from build123d import *

# Parameters (mm, degrees)
EXTRUDE4_DEPTH          = 1.9304
SKETCH2_R               = 0.6604
CUT_EXTRUDE1_DEPTH      = 19.722050478
CIRPATTERN4_COUNT       = 6
CUT_EXTRUDE2_DEPTH      = 12.7
CUT_EXTRUDE2_DEPTH_BACK = 12.7
SKETCH3_R               = 1.397
SKETCH4_R               = 4.445
CUT_EXTRUDE3_DEPTH      = 0.635
SKETCH5_R               = 3.4925
SKETCH5_R_2             = 3.175
EXTRUDE5_DEPTH          = 1.143
RIB10_REACH             = 26.438
SKETCH8_WALL_W          = 52.220152264
SKETCH8_WALL_H          = 0.381
CIRPATTERN5_COUNT       = 8
SKETCH9_R               = 0.79375
SKETCH9_R_2             = 1.1938
CUT_EXTRUDE4_DEPTH      = 25.392925761
CIRPATTERN6_COUNT       = 6
SKETCH10_R              = 5.08
EXTRUDE6_DEPTH          = 0.762
FILLET2_R               = 0.508
SKETCH11_R              = 4.064
EXTRUDE7_DEPTH          = 3.048
FILLET3_R               = 0.889
SKETCH12_R              = 2.8575
CUT_EXTRUDE5_DEPTH      = 3.429
SKETCH14_R              = 1.397
CUT_EXTRUDE6_DEPTH      = 25.557003564
SKETCH15_R              = 0.3175
CUT_EXTRUDE7_DEPTH      = 25.984806887
CIRPATTERN7_COUNT       = 6


with BuildPart() as part:
    # Sketch1 → Extrude4 (new body)
    with BuildSketch(Plane(origin=(0, 0, 0), x_dir=(1, 0, 0), z_dir=(0, 1, 0))):
        with BuildLine():
            Line((5.775220615, -3.829827046), (0, 0))
            Line((0, 0), (5.775220615, 3.829827046))
            Line((5.775220615, 3.829827046), (6.35029977, 3.829827046))
            Line((6.35029977, 3.829827046), (6.35029977, 3.494998084))
            Line((6.35029977, 3.494998084), (15.87469147, 2.35207108))
            ThreePointArc((15.87469147, 2.35207108), (18.22419147, 0.00257108), (15.87469147, -2.34692892))
            Line((15.87469147, -2.34692892), (6.34969147, -3.48992892))
            Line((6.34969147, -3.48992892), (6.34969147, -3.829827046))
            Line((6.34969147, -3.829827046), (5.775220615, -3.829827046))
        make_face()
    extrude4 = extrude(amount=EXTRUDE4_DEPTH)

    # Sketch2 → Cut-Extrude1 (cut, through all)
    with BuildSketch(Plane(origin=(0, 1.9304, 0), x_dir=(-1, 0, 0), z_dir=(0, 1, 0))):
        with Locations((-6.342552501, -4.149920748)):
            Circle(SKETCH2_R)
        with Locations((-6.342552501, 4.149920748)):
            Circle(SKETCH2_R)
    extrude(amount=-CUT_EXTRUDE1_DEPTH, mode=Mode.SUBTRACT)

    # CirPattern4: Extrude4 ×6 about axis
    cirpattern4_axis = Axis((0, 0, 0), (0, 1, 0))
    for i in range(1, CIRPATTERN4_COUNT):
        add(extrude4.rotate(cirpattern4_axis, i * 360 / CIRPATTERN4_COUNT))

    # Sketch3 → Cut-Extrude2 (cut, two sides: drawn at the far end of the back side and taken through both)
    with BuildSketch(Plane(origin=(0, 1.9304, 0), x_dir=(-1, 0, 0), z_dir=(0, 1, 0)).offset(-CUT_EXTRUDE2_DEPTH_BACK)):
        with Locations(Location((0, 0, 0), (0, 0, 90))):
            Circle(SKETCH3_R)
    extrude(amount=CUT_EXTRUDE2_DEPTH + CUT_EXTRUDE2_DEPTH_BACK, mode=Mode.SUBTRACT)

    # Sketch4 → Cut-Extrude3 (cut)
    with BuildSketch(Plane(origin=(0, 1.9304, 0), x_dir=(-1, 0, 0), z_dir=(0, 1, 0))):
        with Locations(Location((0, 0, 0), (0, 0, 90))):
            Circle(SKETCH4_R)
    extrude(amount=-CUT_EXTRUDE3_DEPTH, mode=Mode.SUBTRACT)

    # Sketch5 → Extrude5 (add)
    with BuildSketch(Plane(origin=(0, 1.2954, 0), x_dir=(-1, 0, 0), z_dir=(0, 1, 0))):
        with Locations(Location((0, 0, 0), (0, 0, 90))):
            Circle(SKETCH5_R)
        with Locations(Location((0, 0, 0), (0, 0, 90))):
            Circle(SKETCH5_R_2, mode=Mode.SUBTRACT)
    extrude(amount=EXTRUDE5_DEPTH)

    # Sketch8 wall → Rib10 (add, up to next)
    with BuildSketch(Plane(origin=(-3.967749561, 1.770078976, 0), x_dir=(-0.70753138537, -0.706681921883, 0), z_dir=(0.706681921883, -0.70753138537, 0)), mode=Mode.PRIVATE) as rib10_sk1:
        Rectangle(SKETCH8_WALL_W, SKETCH8_WALL_H)
    rib10_tool1 = extrude(rib10_sk1.sketch, amount=RIB10_REACH, mode=Mode.PRIVATE) - part.part
    rib10 = rib10_tool1.solids().sort_by_distance((-3.967749561, 1.770078976, 0))[0]
    add(rib10)

    # CirPattern5: Rib10 ×8 about axis
    cirpattern5_axis = Axis((0, 0, 0), (0, 1, 0))
    for i in range(1, CIRPATTERN5_COUNT):
        add(rib10.rotate(cirpattern5_axis, i * 360 / CIRPATTERN5_COUNT))

    # Sketch9 → Cut-Extrude4 (cut, through all)
    with BuildSketch(Plane(origin=(0, 1.9304, 0), x_dir=(-1, 0, 0), z_dir=(0, 1, 0))):
        with Locations(Location((7.935119114, 13.749171631, 0), (0, 0, 90))):
            Circle(SKETCH9_R)
        with Locations(Location((5.256324989, 9.107628175, 0), (0, 0, 90))):
            Circle(SKETCH9_R_2)
    cut_extrude4 = extrude(amount=-CUT_EXTRUDE4_DEPTH, mode=Mode.SUBTRACT)

    # CirPattern6: Cut-Extrude4 ×6 about axis
    cirpattern6_axis = Axis((0, 0, 0), (0, 1, 0))
    for i in range(1, CIRPATTERN6_COUNT):
        add(cut_extrude4.rotate(cirpattern6_axis, i * 360 / CIRPATTERN6_COUNT), mode=Mode.SUBTRACT)

    # Sketch10 → Extrude6 (add)
    with BuildSketch(Plane.XZ):
        with Locations(Location((0, 0, 0), (0, 0, 90))):
            Circle(SKETCH10_R)
    extrude(amount=EXTRUDE6_DEPTH)

    # Fillet2
    fillet2_edges = [part.edges().sort_by_distance(p)[0] for p in [
        (0, 0, -5.08),
    ]]
    fillet(fillet2_edges, radius=FILLET2_R)

    # Sketch11 → Extrude7 (add)
    with BuildSketch(Plane.XZ.offset(0.762)):
        with Locations(Location((0, 0, 0), (0, 0, 90))):
            Circle(SKETCH11_R)
    extrude(amount=EXTRUDE7_DEPTH)

    # Fillet3
    fillet3_edges = [part.edges().sort_by_distance(p)[0] for p in [
        (0, -0.762, -4.064),
    ]]
    fillet(fillet3_edges, radius=FILLET3_R)

    # Sketch12 → Cut-Extrude5 (cut)
    with BuildSketch(Plane.XZ.offset(3.81)):
        with Locations(Location((0, 0, 0), (0, 0, 270))):
            Circle(SKETCH12_R)
    extrude(amount=-CUT_EXTRUDE5_DEPTH, mode=Mode.SUBTRACT)

    # Sketch14 → Cut-Extrude6 (cut, through all)
    with BuildSketch(Plane.XZ.offset(0.381)):
        with Locations(Location((0, 0, 0), (0, 0, 90))):
            Circle(SKETCH14_R)
    extrude(amount=-CUT_EXTRUDE6_DEPTH, mode=Mode.SUBTRACT)

    # Sketch15 → Cut-Extrude7 (cut, symmetric)
    with BuildSketch(Plane(origin=(0, 1.9304, 0), x_dir=(-1, 0, 0), z_dir=(0, 1, 0))):
        with Locations((-6.48724684, -3.751940905)):
            Circle(SKETCH15_R)
    cut_extrude7 = extrude(amount=CUT_EXTRUDE7_DEPTH, both=True, mode=Mode.SUBTRACT)

    # CirPattern7: Cut-Extrude7 ×6 about axis
    cirpattern7_axis = Axis((0, 0, 0), (0, 1, 0))
    for i in range(1, CIRPATTERN7_COUNT):
        add(cut_extrude7.rotate(cirpattern7_axis, i * 360 / CIRPATTERN7_COUNT), mode=Mode.SUBTRACT)


solid = part.part
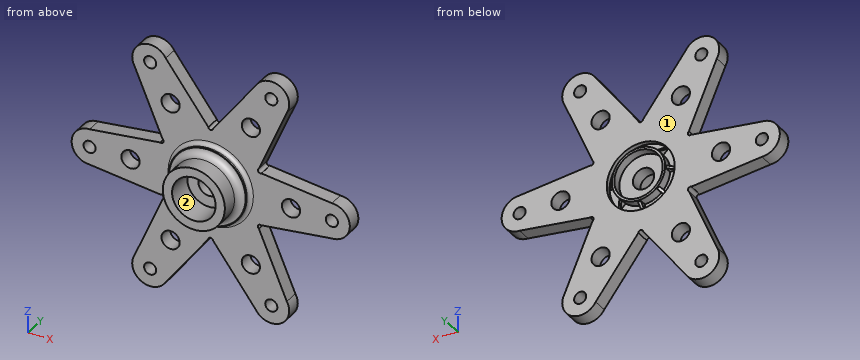
Input: part model. Units: mm. Frame: model coordinates. Face numbers are marked on the shaded views. Coordinates: 2 decimals unless noted, no trailing zeros. Order: outer loops, then holes, each group sorted by start corner. A loop starts at its lowest first (then second) coordinate and runs counter-clockwise, first axis right, second up. Notation, with made-up numbers: M -28.75,39 L -10.75,39 A3 ccw -10.75,44 Z; hole C -30,13 d6. An arc over 180 degrees is marked long. One line per question, with ' | ' between items.
Item 1: Draft query along Z for the marked faces 1 and 2. Return one class per face: released by +Z, released by -Z, zero draft, split by the parting line, or undercut.
Geometry results:
face 1: zero draft | face 2: undercut
Item 2: Pin query (flat end, axial travel): pin 1 (4 mm diameter, centred on x = -10.5, z = -12, fed in from -Y); pin 2 (1.8 mm diameter, centred on x = 7.94, z = 13.75, fed in from +Y); pin 3 (0.8 mm diameter, centred on x = -4, y = 2, fed in from +Z). Return the tip coordinate at first contact, or that it passes through.
Geometry results:
pin 1: stops at y = 0 | pin 2: stops at y = 1.93 | pin 3: stops at z = 12.91
Item 3: Section A-A (y = -2.5). Output: boundary loops of the cut face in (x, z) (1 decimal), then the cut area to 3 significant figures.
Geometry results:
outline: C 0,0 d8.1; hole C 0,0 d5.7 | area: 26.2 mm^2
Item 4: Section C-C (x = 13). Output: boundary loops of the cut face in (y, z).
Geometry results:
outline: M 0,-2.7 L 1.93,-2.7 L 1.93,2.69 L 0,2.69 Z
Item 5: Section B-B (y = 0.75). Give the number of separate pieces and of enclosed holes in the cut face, then the cut area to 3 significant figures.
Geometry results:
separate pieces: 1 | enclosed holes: 13 | area: 480 mm^2
Item 6: Ray query, line 1 along X through (y, z) = (1.5, -13.5); line 2 along Z through (x, y) = (10, 1); line 3 along Y through (x, z) = (7.5, 3). Return the intervals inside material, ascending.
Geometry results:
line 1: x = -10.28 to -8.69, -7.19 to -4.84, 4.83 to 7.18, 8.69 to 10.27 | line 2: z = -14.87 to -12.63, -3.06 to -1.08, 1.08 to 3.05, 12.62 to 14.88 | line 3: y = 0 to 1.93
